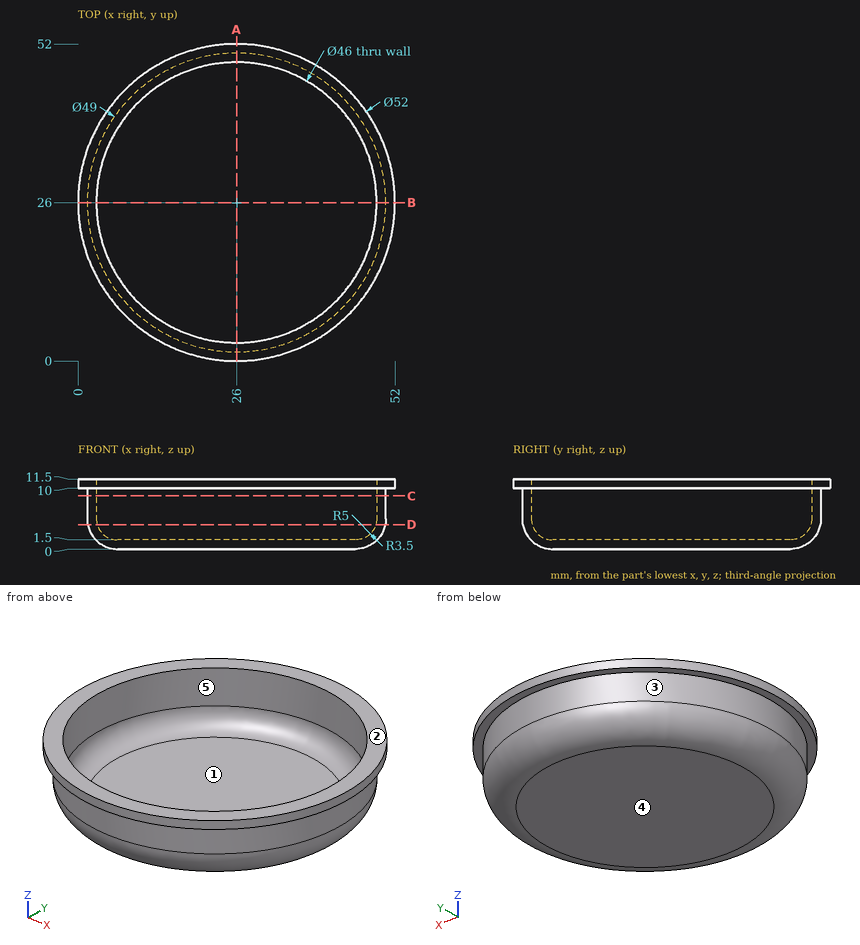
Geometry check sheet. Reference: drawing and pictorial views, mm from the part's lowest x, y, z. A direction names the side the tool comes from. Round coordinates to 2 decimals unless told otherwise and drop trailing zeros. Loops run counter-clockwise (first coordinate to the right, second up) from the corner with the lowest first, then second, coordinate; pieces in that order, holes last. Notation, with made-up numbers: M 62,18 L 90,18 A35 ccw 90,51 Z; hole C 52,82 d1. An arc over 180 degrees is marked long. One line per item, written item: value.
(1) Sectioned sample at D-D, the plane z = 4. Record the cut outline in (x, y).
Computed values:
outline: C 26,26 d48.8; hole C 26,26 d45.71
(2) Release check for a two-part mould opening along Y. For the marked faces 1, 2 and 3 record: +Y half, -Y half, draft (parallel to the pull), parting line (faces both ways), or undercut.
Computed values:
face 1: undercut
face 2: draft
face 3: parting line
(3) Sectioned sample at C-C, the plane z = 8.75. Record the cut outline in (x, y), then the cut area to 3 significant figures.
Computed values:
outline: C 26,26 d49; hole C 26,26 d46
area: 224 mm^2
(4) Thickness scan on line 1 (Z direction, x = 40, y = 35); line 2 (Y direction, x = 26, z = 9.75); line 3 (X direction, y = 17, z = 9). Record the ranges inside material, lowest first.
Computed values:
line 1: z = 0 to 1.5
line 2: y = 1.5 to 3, 49 to 50.5
line 3: x = 3.21 to 4.83, 47.17 to 48.79
(5) Sectioned sample at A-A, the plane x = 26. Record the cut outline in (y, z).
Computed values:
outline: M 0,10 L 1.5,10 L 1.5,5 A5 ccw 6.5,0 L 45.5,0 A5 ccw 50.5,5 L 50.5,10 L 52,10 L 52,11.5 L 49,11.5 L 49,5 A3.5 cw 45.5,1.5 L 6.5,1.5 A3.5 cw 3,5 L 3,11.5 L 0,11.5 Z
(6) Access from +Z, -Z, +X, -X, +Y, -Y to the whole of each face (thin tool, end or side, straight path). Record for the marked faces 4 and 5.
Computed values:
face 4: -Z, +X, -X, +Y, -Y
face 5: +Z
(7) Depth check by flat-ended pin: pin 1 Ø5 at (x, z) = (42.5, 1) entering from +Y; pin 2 Ø5 at (x, y) = (5.5, 37) entering from -Z; pin 3 Ø11.5 at (x, y) = (21, 20.5) entering from +Z. Enter the tip coordinate at first touch or a pass-through.
Computed values:
pin 1: stops at y = 44.92
pin 2: stops at z = 0.16
pin 3: stops at z = 1.5
